Here's how the part is built. I have some questions about the finished solid (model axes, mm). Face numbers are marked on the shaded views. A direction names the side the tool comes from. Coordinates: 2 decimals unless noted, no trailing zeros. Write each loop counter-clockwise with the first axis right and the second up, starting at its lowest first coordinate (ties: lowest second). Pieces come first, ordered by that corner, then holes. Notation, with made-up numbers: M 18.5,83.5 L 47.5,83.5 A24 ccw 47.5,122.5 Z; hole C 84.5,25 d6. An arc over 180 degrees is marked long. Use one line per item in the form item = value. Start each with the question number.
1. I want a section at C-C, the plane z = 4.5. List the corners of the cut face in (x, y) for me, plus the area to 3 significant figures.
2. On a 3-axis mill with a long thin cutter (end or side, diameter ignored), from which of +Z, -Z, +X, -X, +Y, -Y can I reach the whole of each face in a straight line? I mean the marked faces 1 and 2. Say none if no direction works.
3. I want a section at A-A, the plane y = 0. List the corners of the cut face in (x, z) for me, plus the area to 3 significant figures.
4. I want a section at D-D, the plane z = 9. List the corners of the cut face in (x, y) for me.
5. Please list where these lines run through material, in increasing order: line 1 along Y through (x, z) = (0, 1.6); line 2 along Z through (x, y) = (-5.25, 17); line 3 along Z through (x, y) = (-9, -3). Write a range as [from, to].
6. I'm going to push flat-ended pins straight in: pin 1 Ø5 at (y, z) = (9.5, 5) entering from +X; pin 2 Ø1.5 at (y, z) = (-0.5, 9) entering from +X; pin 3 Ø5 at (x, y) = (-1.5, -12) entering from +Z. Where does each tip first touch, or does it pass through?
7. I want a section at B-B, the plane x = 0. List the corners of the cut face in (y, z) for me, plus the area to 3 significant figures.
8. Thinking about a two-plate mould opening in X: for the marked faces 3, 4, 5 and 6, which applies, released by +X, released by -X, zero draft, split by the parting line, or undercut?
from build123d import *

# Parameters (mm, degrees)
CROQUIS1_R              = 4
CROQUIS1_R_2            = 2.6
SALIENTE_EXTRUIR1_DEPTH = 7
CROQUIS2_R              = 2.6
CORTAR_EXTRUIR1_DEPTH   = 5
CROQUIS3_R              = 7.25
CROQUIS3_R_2            = 4
SALIENTE_EXTRUIR2_DEPTH = 6


with BuildPart() as part:
    # Croquis1 → Saliente-Extruir1 (new body)
    with BuildSketch(Plane.XY):
        with BuildLine():
            Line((10.288824315, -3.891027397), (4.514634908, -19.880359362))
            ThreePointArc((4.514634908, -19.880359362), (0, -23.05), (-4.514634908, -19.880359362))
            Line((-4.514634908, -19.880359362), (-10.288824315, -3.891027397))
            ThreePointArc((-10.288824315, -3.891027397), (-11, 0), (-10.288824315, 3.891027397))
            Line((-10.288824315, 3.891027397), (-4.514634908, 19.880359362))
            ThreePointArc((-4.514634908, 19.880359362), (0, 23.05), (4.514634908, 19.880359362))
            Line((4.514634908, 19.880359362), (10.288824315, 3.891027397))
            ThreePointArc((10.288824315, 3.891027397), (11, 0), (10.288824315, -3.891027397))
        make_face()
        Circle(CROQUIS1_R, mode=Mode.SUBTRACT)
        with Locations((0, 18.25)):
            Circle(CROQUIS1_R_2, mode=Mode.SUBTRACT)
        with Locations((0, -18.25)):
            Circle(CROQUIS1_R_2, mode=Mode.SUBTRACT)
    extrude(amount=SALIENTE_EXTRUIR1_DEPTH)

    # Croquis2 → Cortar-Extruir1 (cut)
    with BuildSketch(Plane.XY.offset(7)):
        with BuildLine():
            Line((-4.514634908, 19.880359362), (-10.288824315, 3.891027397))
            ThreePointArc((-10.288824315, 3.891027397), (0, 11), (10.288824315, 3.891027397))
            Line((10.288824315, 3.891027397), (4.514634908, 19.880359362))
            ThreePointArc((4.514634908, 19.880359362), (0, 23.05), (-4.514634908, 19.880359362))
        make_face()
        with Locations((0, 18.25)):
            Circle(CROQUIS2_R, mode=Mode.SUBTRACT)
        with BuildLine():
            ThreePointArc((10.288824315, -3.891027397), (0, -11), (-10.288824315, -3.891027397))
            Line((-10.288824315, -3.891027397), (-4.514634908, -19.880359362))
            ThreePointArc((-4.514634908, -19.880359362), (0, -23.05), (4.514634908, -19.880359362))
            Line((4.514634908, -19.880359362), (10.288824315, -3.891027397))
        make_face()
        with Locations((0, -18.25)):
            Circle(CROQUIS2_R, mode=Mode.SUBTRACT)
    extrude(amount=-CORTAR_EXTRUIR1_DEPTH, mode=Mode.SUBTRACT)

    # Croquis3 → Saliente-Extruir2 (add)
    with BuildSketch(Plane.XY.offset(7)):
        Circle(CROQUIS3_R)
        Circle(CROQUIS3_R_2, mode=Mode.SUBTRACT)
    extrude(amount=SALIENTE_EXTRUIR2_DEPTH)


solid = part.part
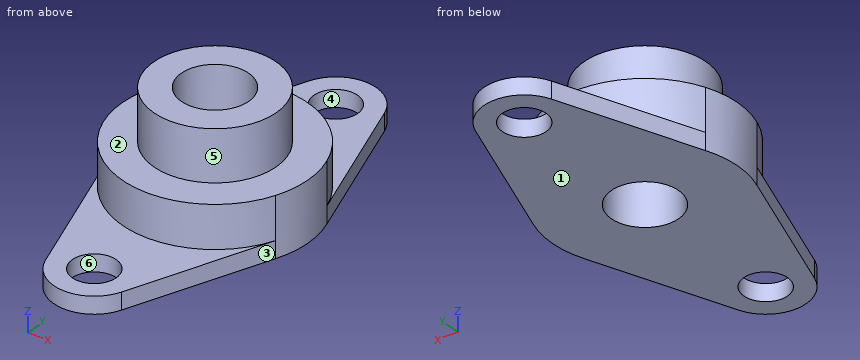
Answer list:
q1.outline = C 0,0 d22; hole C 0,0 d8
q1.area = 330 mm²
q2.face_1 = -Z, +X, -X, +Y, -Y
q2.face_2 = +Z
q3.outline = M -11,0 L -4,0 L -4,13 L -7.25,13 L -7.25,7 L -11,7 Z; M 4,0 L 11,0 L 11,7 L 7.25,7 L 7.25,13 L 4,13 Z
q3.area = 137 mm²
q4.outline = C 0,0 d14.5; hole C 0,0 d8
q5.line_1 = [-23.05, -20.85], [-15.65, -4], [4, 15.65], [20.85, 23.05]
q5.line_2 = [0, 2]
q5.line_3 = [0, 7]
q6.pin_1 = 8.49
q6.pin_2 = 7.25
q6.pin_3 = 7
q7.outline = M -23.05,0 L -20.85,0 L -20.85,2 L -23.05,2 Z; M -15.65,0 L -4,0 L -4,13 L -7.25,13 L -7.25,7 L -11,7 L -11,2 L -15.65,2 Z; M 4,0 L 15.65,0 L 15.65,2 L 11,2 L 11,7 L 7.25,7 L 7.25,13 L 4,13 Z; M 20.85,0 L 23.05,0 L 23.05,2 L 20.85,2 Z
q7.area = 164 mm²
q8.face_3 = released by +X
q8.face_4 = undercut
q8.face_5 = split by the parting line
q8.face_6 = undercut
